The model under review builds one solid part; all positions refer to its coordinate system, in mm. A direction names the side the tool comes from. Round coordinates to 2 decimals unless told otherwise and drop trailing zeros. Order: outer loops, then holes, each group sorted by start corner. A loop starts at its lowest first (then second) coordinate and runs counter-clockwise, first axis right, second up. Notation, with made-up numbers: M 3,76 L 15,76 A16 ccw 15,89 Z; hole C -27,16.25 d4. An arc over 180 degrees is marked long. Answer as a JSON object with one key per item and string values. Group by question number.
1. Add section B-B on x = 7. State the section outline as (y, z) points, and give its area (3 significant figures).
2. Machinability: for faces 4 (the face through (-15.9, 0, 105)), 5 (the face through (17.5, 0, 212)), which of the approach directions +Z, -Z, +X, -X, +Y, -Y give a long, thin tool a straight path to every point of the face, cutting with its end or side? Answer none if there is none.
3. Add section C-C on x = -10. State the section outline as (y, z) points.
4. Mouldability with a two-part tool opening along Y and no side actions: class faces 1 (the face through (3, 15.9, 212)), 2 (the face through (-17.5, 0, 106)), 3 (the face through (0.2, -17.5, 211.8)) as released by +Y, released by -Y, zero draft, split by the parting line, or undercut.
5. Add section D-D on z = 395. State the section outline as (x, y) points, and give its area (3 significant figures).
6. To check wall thickness, follow probe 1 along Y at (x, z) = (-6.5, 159); probe 2 along X at (y, z) = (-15.5, 70). State the ranges of each line that lie inside material, in increasing order. Write a range as [from, to].
7. Add section A-A on y = 9.5. State the section outline as (x, z) points.
8. Clearance check with flat-ended pins moving along their axes: P1, Ø0.5, axis at x = -16.5, y = -7, coming from the -Z side; P2, Ø1.8, axis at y = 17, z = 218.5, coming from the -X side; P3, Ø1.8, axis at x = -16.5, y = -5.5, coming from the +Z side. State where each tip first meets the part, or that it passes through.
Autodesk Inventor part; units mm, degrees
ref_plane "Start plane" through (0, 0, -17.5) normal (0, 0, 1) x (1, 0, 0)
ref_plane "End plane" through (0, 0, 447.5) normal (0, 0, 1) x (1, 0, 0)
ref_plane "Work Plane4" through (17.5, 0, 447.5) normal (-0.7071, 0, 0.7071) x (0.7071, 0, 0.7071)
ref_plane "Start plane" through (0, 0, -17.5) normal (0, 0, 1) x (1, 0, 0)
ref_plane "End plane" through (0, 0, 447.5) normal (0, 0, 1) x (1, 0, 0)
sketch "Sketch" plane through (0, 0, 0) normal (0, 0, 1) x (1, 0, 0)
  line L0 (-17.5, -14.3) -> (-17.5, 14.3)
  line L1 (-14.3, 17.5) -> (14.3, 17.5)
  line L2 (17.5, 14.3) -> (17.5, -14.3)
  line L3 (14.3, -17.5) -> (-14.3, -17.5)
  arc A0 (-17.5, -14.3) -> (-14.3, -17.5) centre (-14.3, -14.3) ccw
  arc A1 (-14.3, 17.5) -> (-17.5, 14.3) centre (-14.3, 14.3) ccw
  arc A2 (17.5, 14.3) -> (14.3, 17.5) centre (14.3, 14.3) ccw
  arc A3 (14.3, -17.5) -> (17.5, -14.3) centre (14.3, -14.3) ccw
  arc A4 (-14.3, 15.9) -> (-15.9, 14.3) centre (-14.3, 14.3) ccw
  line L4 (-14.3, 15.9) -> (14.3, 15.9)
  arc A5 (15.9, 14.3) -> (14.3, 15.9) centre (14.3, 14.3) ccw
  line L5 (15.9, 14.3) -> (15.9, -14.3)
  arc A6 (14.3, -15.9) -> (15.9, -14.3) centre (14.3, -14.3) ccw
  line L6 (14.3, -15.9) -> (-14.3, -15.9)
  arc A7 (-15.9, -14.3) -> (-14.3, -15.9) centre (-14.3, -14.3) ccw
  line L7 (-15.9, -14.3) -> (-15.9, 14.3)
  line L8 (0, 25.4278) -> (0, -25.4278) construction
  line L9 (-25.4278, 0) -> (25.4278, 0) construction
  dimension "d7" = 3.2
  dimension "d10" = 35
  dimension "d11" = 35
  dimension "d12" = 1.6
  dimension "d15" = 17.5
  dimension "d16" = 17.5
extrude "Body" add sketch "Sketch" along normal up to surface (465 mm away) from surface at -17.5
sketch "Sketch3" plane through (0, 0, 0) normal (0, 0, 1) x (1, 0, 0)
  line L0 (0, 0) -> (10, 0)
ref_plane "Work Plane3" through (0, 0, 0) normal (0, -1, 0) x (1, 0, 0)
sketch "Sketch4" plane through (0, 0, 0) normal (0, -1, 0) x (1, 0, 0)
  line L0 (-2, -17.5) -> (12, -17.5)
  line L1 (-2, 447.5) -> (12, 447.5)
  dimension "d18" = 465
ref_plane "Work Plane4" through (17.5, 0, 447.5) normal (-0.7071, 0, 0.7071) x (0.7071, 0, 0.7071)
split "Split1" plane through (17.5, 0, 447.5) removes the side toward (-0.7071, 0, 0.7071)
ref_plane "Work Plane5" through (17.5, 0, -17.5) normal (-0.7071, 0, -0.7071) x (-0.7071, 0, 0.7071)
split "Split2" plane through (17.5, 0, -17.5) removes the side toward (-0.7071, 0, -0.7071)
ref_plane "Work Plane6" through (-730, 0, 215) normal (1, 0, 0) x (0, 0, -1)
ref_plane "Work Plane7" through (0, 0, 215) normal (1, 0, 0) x (0, 0, -1)
ref_plane "Work Plane8" through (-365, 0, 215) normal (1, 0, 0) x (0, 0, -1)
sketch "Sketch5" plane through (-365, 0, 215) normal (1, 0, 0) x (0, 0, -1)
  arc A0 (-17.5, -14.3) -> (-14.3, -17.5) centre (-14.3, -14.3) ccw
  line L0 (-17.5, -14.3) -> (-17.5, 14.3)
  arc A1 (-14.3, 17.5) -> (-17.5, 14.3) centre (-14.3, 14.3) ccw
  line L1 (-14.3, 17.5) -> (14.3, 17.5)
  arc A2 (17.5, 14.3) -> (14.3, 17.5) centre (14.3, 14.3) ccw
  line L2 (17.5, 14.3) -> (17.5, -14.3)
  arc A3 (14.3, -17.5) -> (17.5, -14.3) centre (14.3, -14.3) ccw
  line L3 (14.3, -17.5) -> (-14.3, -17.5)
  arc A4 (-14.3, 15.9) -> (-15.9, 14.3) centre (-14.3, 14.3) ccw
  line L4 (-14.3, 15.9) -> (14.3, 15.9)
  arc A5 (15.9, 14.3) -> (14.3, 15.9) centre (14.3, 14.3) ccw
  line L5 (15.9, 14.3) -> (15.9, -14.3)
  arc A6 (14.3, -15.9) -> (15.9, -14.3) centre (14.3, -14.3) ccw
  line L6 (14.3, -15.9) -> (-14.3, -15.9)
  arc A7 (-15.9, -14.3) -> (-14.3, -15.9) centre (-14.3, -14.3) ccw
  line L7 (-15.9, -14.3) -> (-15.9, 14.3)
extrude "Extrusion2" cut sketch "Sketch5" along normal up to surface (730 mm away) from surface at -365 contours L0 A1 L1 A2 L2 A3 L3 A0 | L4 A5 L5 A6 L6 A7 L7 A4
equation "\"d7\" = G_IR"
equation "\"d10\" = G_H"
equation "\"d11\" = G_W"
equation "\"d12\" = G_T"
equation "\"d15\" = 0.5 * d10"
equation "\"d16\" = 0.5 * d11"
equation "\"d3\" = G_L"
equation "\"G_W\" = 35"
equation "\"G_H\" = 35"
equation "\"G_T\" = 1.6"
equation "\"G_IR\" = 3.2"
equation "\"G_L\" = d18"
equation "\"G_OFFSET_START\" = 17.5"
equation "\"G_OFFSET_END\" = 17.5"
equation "\"d13\" = -G_OFFSET_START"
equation "\"d14\" = G_OFFSET_END + B_L"
properties part number "AS 1163 - C350L0 35x35x1.6 SHS - 465" material "Steel, Mild"
Recorded:
{
 "1": {"outline": "M -17.5,-7 L -15.9,-7 L -15.9,437 L -17.5,437 Z; M 15.9,-7 L 17.5,-7 L 17.5,437 L 15.9,437 Z", "area": "1,420 mm²"},
 "2": {"face 4": "+Z, -Z", "face 5": "+Z, -Z, +X, +Y, -Y"},
 "3": {"outline": "M -17.5,10 L -15.9,10 L -15.9,197.93 A3.2 cw -17.5,200.7 Z; M -17.5,229.3 A3.2 cw -15.9,232.07 L -15.9,420 L -17.5,420 Z; M 15.9,10 L 17.5,10 L 17.5,200.7 A3.2 cw 15.9,197.93 Z; M 15.9,232.07 A3.2 cw 17.5,229.3 L 17.5,420 L 15.9,420 Z"},
 "4": {"face 1": "undercut", "face 2": "zero draft", "face 3": "released by -Y"},
 "5": {"outline": "M -17.5,-14.3 A3.2 ccw -14.3,-17.5 L 14.3,-17.5 A3.2 ccw 17.5,-14.3 L 17.5,14.3 A3.2 ccw 14.3,17.5 L -14.3,17.5 A3.2 ccw -17.5,14.3 Z; hole M -15.9,-14.3 A1.6 ccw -14.3,-15.9 L 14.3,-15.9 A1.6 ccw 15.9,-14.3 L 15.9,14.3 A1.6 ccw 14.3,15.9 L -14.3,15.9 A1.6 ccw -15.9,14.3 Z", "area": "207 mm²"},
 "6": {"probe 1": "y = [-17.5, -15.9], [15.9, 17.5]", "probe 2": "x = [-17.27, -15.36], [15.36, 17.27]"},
 "7": {"outline": "M -17.5,17.5 L -15.9,15.9 L -15.9,197.5 L -17.5,197.5 Z; M -17.5,232.5 L -15.9,232.5 L -15.9,414.1 L -17.5,412.5 Z; M 15.9,-15.9 L 17.5,-17.5 L 17.5,447.5 L 15.9,445.9 Z"},
 "8": {"P1": "stops at z = 16.25", "P2": "stops at x = 0", "P3": "stops at z = 414.1"}
}
